```python
from build123d import *

# Parameters (mm, degrees)
BOSS_EXTRUDE1_DEPTH = 5


with BuildPart() as part:
    # Sketch1 → Boss-Extrude1 (new body)
    with BuildSketch(Plane(origin=(0, 0, 0), x_dir=(0, 0, -1), z_dir=(1, 0, 0))):
        with BuildLine():
            Line((6.35, 17.292870535), (6.35, 19.05))
            Line((6.35, 19.05), (0, 19.05))
            Line((0, 19.05), (0, 0))
            Line((0, 0), (6.35, 0))
            Line((6.35, 0), (6.35, 13.292870535))
            ThreePointArc((6.35, 13.292870535), (4.35, 15.292870535), (6.35, 17.292870535))
        make_face()
        with BuildLine():
            Line((12.7, 19.05), (6.35, 19.05))
            Line((6.35, 19.05), (6.35, 17.292870535))
            ThreePointArc((6.35, 17.292870535), (7.764213562, 16.707084098), (8.35, 15.292870535))
            ThreePointArc((8.35, 15.292870535), (7.764213562, 13.878656973), (6.35, 13.292870535))
            Line((6.35, 13.292870535), (6.35, 0))
            Line((6.35, 0), (12.7, 0))
            Line((12.7, 0), (12.7, 19.05))
        make_face()
    extrude(amount=BOSS_EXTRUDE1_DEPTH)


solid = part.part
```
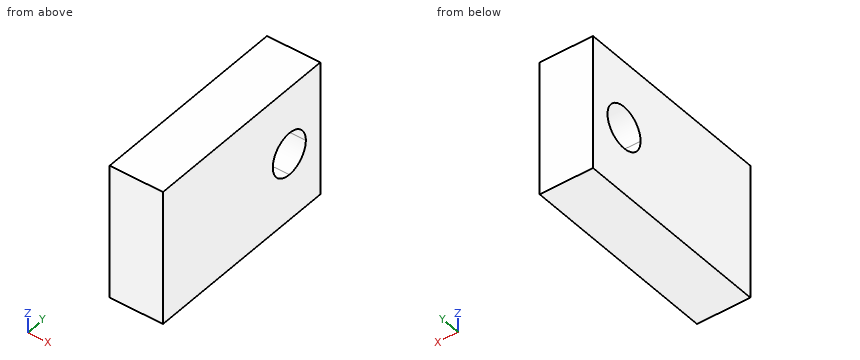
The listing builds one solid part. Answer for the finished solid, in the listing's coordinates (mm). Round coordinates to 2 decimals unless told otherwise and drop trailing zeros. Write each loop counter-clockwise with the first axis right and the second up, starting at its lowest first coordinate (ties: lowest second). Pieces come first, ordered by that corner, then holes. Notation, with made-up numbers: (8.5, -19.5) -> (12.5, -19.5) arc R14 ccw to (12.5, -9.5) -> close; hole circle Ø2 at (-29, -38). An arc over 180 degrees is marked (long way). Answer as a JSON object with one key per item and string values. Group by question number.
Q1. Section A-A (z = -5.75) is taken. Write down the section's boundary in (x, y) (3 decimals).
Q2. Section B-B (x = 1.15) is taken. Write down the section's boundary in (y, z), plus the area to 3 significant figures.
Q3. This flat-tipped pin is pushed along its axis until it touches: pin 1 Ø1 at (x, z) = (2, -3.5) entering from -Y. Where does it stop, or does it pass through?
Q4. Straight lines are drawn through the part: line 1 along Y through (x, z) = (4.3, -6.25); line 2 along Z through (x, y) = (0.95, 15.25); line 3 along Y through (x, z) = (3, -7). For each, find the intervals that lie inside material, in ascending order.
Check values:
{
 "1": {"outline": "(0, 0) -> (5, 0) -> (5, 13.385) -> (0, 13.385) -> close; (0, 17.201) -> (5, 17.201) -> (5, 19.05) -> (0, 19.05) -> close"},
 "2": {"outline": "(0, -12.7) -> (19.05, -12.7) -> (19.05, 0) -> (0, 0) -> close; hole circle Ø4 at (15.29, -6.35)", "area": "229 mm^2"},
 "3": {"pin 1": "y = 0"},
 "4": {"line 1": "0 to 13.3, 17.29 to 19.05", "line 2": "-12.7 to -8.35, -4.35 to 0", "line 3": "0 to 13.4, 17.18 to 19.05"}
}
